```python
from build123d import *

# Parameters (mm, degrees)
SKETCH_1_R               = 28.35
EXTRUDE_1_DEPTH          = 6
SKETCH_2_R               = 16
EXTRUDE_2_DEPTH          = 12
SKETCH_3_R               = 6.5
CUT_EXTRUDE_1_DEPTH      = 44.948208155
HOLE_WIZARD_M5_2_D       = 4.2
PATTERN_CIRCULAR_1_COUNT = 6
CUT_EXTRUDE_3_REACH      = 57.63
CUT_EXTRUDE_3_END_RADIUS = 6.5
SKETCH_6_R               = 2.1
PATTERN_CIRCULAR_2_COUNT = 2
PATTERN_CIRCULAR_2_ANGLE = 90


with BuildPart() as part:
    # 草圖1 → 填料-伸長1 (new body)
    with BuildSketch(Plane.XY):
        Circle(SKETCH_1_R)
    extrude(amount=EXTRUDE_1_DEPTH)

    # 草圖2 → 填料-伸長2 (add)
    with BuildSketch(Plane.XY.offset(6)):
        Circle(SKETCH_2_R)
    extrude(amount=EXTRUDE_2_DEPTH)

    # 草圖3 → 除料-伸長1 (cut, through all)
    with BuildSketch(Plane.XY.offset(18)):
        Circle(SKETCH_3_R)
    extrude(amount=-CUT_EXTRUDE_1_DEPTH, mode=Mode.SUBTRACT)

    # M5 螺紋孔2 (through all)
    with Locations(Plane(origin=(0, 0, 0), x_dir=(-1, 0, 0), z_dir=(0, 0, -1))):
        with Locations((0, 23.75)):
            hole_wizard_m5_2 = Hole(HOLE_WIZARD_M5_2_D / 2)

    # 環狀複製排列1: M5 螺紋孔2 ×6 about axis
    pattern_circular_1_axis = Axis((0, 0, 0), (0, 0, 1))
    for i in range(1, PATTERN_CIRCULAR_1_COUNT):
        add(hole_wizard_m5_2.rotate(pattern_circular_1_axis, i * 360 / PATTERN_CIRCULAR_1_COUNT), mode=Mode.SUBTRACT)

    # 除料-伸長3: up to this cylinder (the profile starts outside it)
    cut_extrude_3_end = Plane(origin=(0, 0, 11), z_dir=(0, 0, 1)) * Cylinder(CUT_EXTRUDE_3_END_RADIUS, 129.26, mode=Mode.PRIVATE)
    # 草圖6 → 除料-伸長3 (cut, up to the surface)
    with BuildSketch(Plane(origin=(16, 0, 0), x_dir=(0, 0, -1), z_dir=(1, 0, 0)), mode=Mode.PRIVATE) as cut_extrude_3_sk1:
        with Locations((-11, 0)):
            Circle(SKETCH_6_R)
    cut_extrude_3_tool1 = extrude(cut_extrude_3_sk1.sketch, amount=-CUT_EXTRUDE_3_REACH, mode=Mode.PRIVATE) - cut_extrude_3_end
    cut_extrude_3 = cut_extrude_3_tool1.solids().sort_by_distance((16, 0, 11))[0]
    add(cut_extrude_3, mode=Mode.SUBTRACT)

    # 環狀複製排列2: 除料-伸長3 ×2 about axis
    pattern_circular_2_axis = Axis((0, 0, 18), (0, 0, 1))
    for i in range(1, PATTERN_CIRCULAR_2_COUNT):
        add(cut_extrude_3.rotate(pattern_circular_2_axis, i * PATTERN_CIRCULAR_2_ANGLE / (PATTERN_CIRCULAR_2_COUNT - 1)), mode=Mode.SUBTRACT)


solid = part.part
```
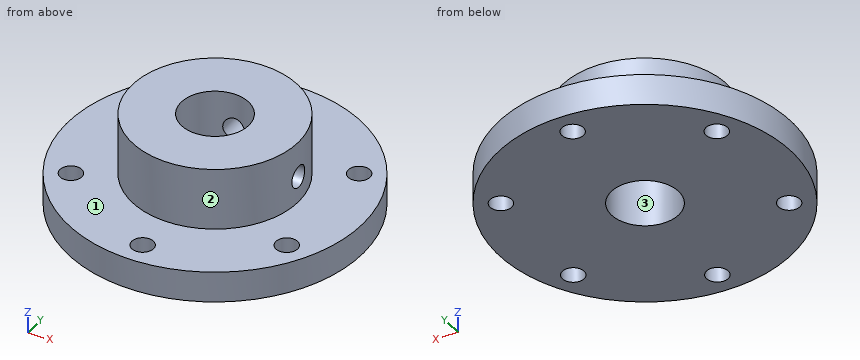
Verification items for the finished model (mm, model axes). Face numbers are marked on the shaded views. Round coordinates to 2 decimals unless told otherwise and drop trailing zeros. Write each loop counter-clockwise with the first axis right and the second up, starting at its lowest first coordinate (ties: lowest second). Pieces come first, ordered by that corner, then holes.
1. Gauge pin test, flat ends, axial feed: P1, Ø4, axis at x = 0, y = 23.75, coming from the -Z side; P2, Ø1.5, axis at x = -4, y = -22.5, coming from the +Z side; P3, Ø6.5, axis at x = 0, z = 11, coming from the -Y side; P4, Ø2, axis at x = -3, z = 9.5, coming from the +Y side. Record the tip position at first contact, or that the pin passes through.
2. Scan lines: L1, parallel to Y at x = -19, z = 5; L2, parallel to X at y = -11, z = 5.25; L3, parallel to Z at x = -19, y = 2. Record each from-to range of solid material in increasing order.
3. Draft check along X on the marked faces 1, 2 and 3. Enter one of: +X half, -X half, draft (parallel to the pull), parting line (faces both ways), or undercut.
4. Section check A-A on y = 0. Enter the section's corners in (x, z).
5. Section check C-C on x = 9.5. Enter the section's corners in (y, z), plus the area to 3 significant figures.
6. Section check B-B on z = 11. Enter the section's corners in (x, y).
7. Section check D-D on y = 23.75. Enter the section's corners in (x, z).
Answer:
1. P1: passes through
1. P2: stops at z = 6
1. P3: stops at y = -16
1. P4: stops at y = 15.87
2. L1: y = -21.04 to -13.27, -10.48 to 10.48, 13.27 to 21.04
2. L2: x = -26.13 to -22.48, -18.66 to 18.66, 22.48 to 26.13
2. L3: z = 0 to 6
3. face 1: draft
3. face 2: parting line
3. face 3: undercut
4. outline: (-28.35, 0) - (-6.5, 0) - (-6.5, 18) - (-16, 18) - (-16, 6) - (-28.35, 6) - close; (6.5, 0) - (28.35, 0) - (28.35, 6) - (16, 6) - (16, 8.9) - (6.5, 8.9) - close; (6.5, 13.1) - (16, 13.1) - (16, 18) - (6.5, 18) - close
5. outline: (-26.71, 0) - (26.71, 0) - (26.71, 6) - (12.87, 6) - (12.87, 18) - (-12.87, 18) - (-12.87, 6) - (-26.71, 6) - close; hole circle Ø4.2 at (0, 11)
5. area: 616 mm2
6. outline: (-2.1, 6.15) - (-2.1, 15.86) arc R16 ccw (long way) to (15.86, -2.1) - (6.15, -2.1) arc R6.5 cw (long way) to start; (2.1, 6.15) arc R6.5 cw to (6.15, 2.1) - (15.86, 2.1) arc R16 ccw to (2.1, 15.86) - close
7. outline: (-15.48, 0) - (-2.1, 0) - (-2.1, 6) - (-15.48, 6) - close; (2.1, 0) - (15.48, 0) - (15.48, 6) - (2.1, 6) - close
